```python
from build123d import *

# Parameters (mm, degrees)
EXTRUDE001_DEPTH = 3
FILLET_R         = 1
SKETCH_W         = 40
SKETCH_H         = 40
EXTRUDE_DEPTH    = 140
SKETCH008_R      = 1
EXTRUDE007_DEPTH = 10
EXTRUDE006_DEPTH = 5
EXTRUDE005_DEPTH = 5


with BuildPart() as fillet_body:
    # Sketch001 → Extrude001 (new body)
    with BuildSketch(Plane.XY.offset(-140)):
        with BuildLine():
            Line((0, -2), (40, -2))
            ThreePointArc((40, -2), (41.414214, -1.414214), (42, 0))
            Line((42, 0), (42, 40))
            ThreePointArc((42, 40), (41.414214, 41.414214), (40, 42))
            Line((40, 42), (0, 42))
            ThreePointArc((0, 42), (-1.414214, 41.414214), (-2, 40))
            Line((-2, 40), (-2, 0))
            ThreePointArc((-2, 0), (-1.414214, -1.414214), (0, -2))
        make_face()
    extrude(amount=-EXTRUDE001_DEPTH)

    # Fillet
    fillet_edges = [fillet_body.edges().sort_by_distance(p)[0] for p in [
        (20, 42, -143),
        (-1.414214, 41.414214, -143),
        (-2, 20, -143),
    ]]
    fillet(fillet_edges, radius=FILLET_R)


with BuildPart() as fusion:
    # Sketch → Extrude (new body)
    with BuildSketch(Plane.XY):
        with BuildLine():
            Line((0, -2), (40, -2))
            ThreePointArc((40, -2), (41.414214, -1.414214), (42, 0))
            Line((42, 0), (42, 40))
            ThreePointArc((42, 40), (41.414214, 41.414214), (40, 42))
            Line((40, 42), (0, 42))
            ThreePointArc((0, 42), (-1.414214, 41.414214), (-2, 40))
            Line((-2, 40), (-2, 0))
            ThreePointArc((-2, 0), (-1.414214, -1.414214), (0, -2))
        make_face()
        with Locations((20, 20)):
            Rectangle(SKETCH_W, SKETCH_H, mode=Mode.SUBTRACT)
    extrude(amount=-EXTRUDE_DEPTH)

    # Fusion: union Fillet body
    add(fillet_body.part)


with BuildPart() as extrude007:
    # Sketch008 → Extrude007 (new body)
    with BuildSketch(Plane.XY):
        with Locations((2, 38)):
            Circle(SKETCH008_R)
        with Locations((38, 38)):
            Circle(SKETCH008_R)
        with Locations((20, 2)):
            Circle(SKETCH008_R)
    extrude(amount=-EXTRUDE007_DEPTH)


with BuildPart() as extrude006:
    # Sketch010 → Extrude006 (new body)
    with BuildSketch(Plane.YZ.offset(17.5)):
        Polygon((0, 0), (5, 0), (0, -10), align=None)
    extrude(amount=EXTRUDE006_DEPTH)


with BuildPart() as fusion004:
    # Sketch009 → Extrude005 (new body)
    with BuildSketch(Plane.XZ.offset(-40)):
        Polygon((0, 0), (5, 0), (0, -10), align=None)
        Polygon((40, 0), (35, 0), (40, -10), align=None)
    extrude(amount=EXTRUDE005_DEPTH)

    # Fusion003: union Extrude006
    add(extrude006.part)

    # Cut: cut Extrude007
    add(extrude007.part, mode=Mode.SUBTRACT)


with BuildPart() as fusion004_1:
    # Cut placement: moved
    add(fusion004.part.moved(Location((0, 0, -2))))

    # Fusion004: union Fusion
    add(fusion.part)


solid = fusion004_1.part
```
Could you check a few things on this model? Use its own coordinates, in mm. A direction names the side the tool comes from. Coordinates: 2 decimals unless noted, no trailing zeros. Order: outer loops, then holes, each group sorted by start corner. A loop starts at its lowest first (then second) coordinate and runs counter-clockwise, first axis right, second up. Notation, with made-up numbers: M -35.75,68.25 L 13.25,68.25 A27 cw 13.25,95.25 Z; hole C 37,78 d5. An arc over 180 degrees is marked long. Use a Markdown table: item, result. Add a question column.
Q1. I'm going to push flat-ended pins straight in: pin 1 (3 mm diameter, centred on x = 28, y = 22, fed in from +Z); pin 2 (20 mm diameter, centred on x = 28, y = 29.5, fed in from +Z). Where does each tip first touch, or does it pass through?
Q2. Which directions (+Z, -Z, +X, -X, +Y, -Y) give clear straight access to the entire face, cutting with the end or side of a thin tool? Please do faces 1 (the flat face through (2.535, 36.979, -6.93)), 2 (the flat face through (20, -2, -70)), 3 (the flat face through (3, 37, -2)).
Q3. I want a section at B-B on z = -94.5. List the corners of the cut face in (x, y) for me, then the cut area to 3 significant figures.
Q4. If I drill on L1, parallel to Y at x = 38, z = -5.5; L2, parallel to X at y = 38, z = -7; L3, parallel to Y at x = 11, z = -88, over which ranges is the centre line in solid material (lowest first)?
Q5. I want a section at A-A on y = 19. List the corners of the cut face in (x, z) for me, then the cut area to 3 significant figures.
Q6. We'd pull the mould along X, two halves only. Please class faces 4 (the flat face through (18.854, 2.535, -6.93)), 5 (the flat face through (-2, 20, -70)), 6 (the flat face through (20, 42, -70)): pulls with the +X half, pulls with the -X half, needs draft (parallel to the pull), parting line crosses it, or undercut.
Checked values:
| question | item | result |
|---|---|---|
| 1 | pin 1 | z = -140 |
| 1 | pin 2 | z = -2 |
| 2 | face 1 | none |
| 2 | face 2 | +Z, -Z, +X, -X, -Y |
| 2 | face 3 | +Z |
| 3 | outline | M -2,0 A2 ccw 0,-2 L 40,-2 A2 ccw 42,0 L 42,40 A2 ccw 40,42 L 0,42 A2 ccw -2,40 Z; hole M 0,0 L 40,0 L 40,40 L 0,40 Z |
| 3 | area | 333 mm² |
| 4 | L1 | -2 to 0, 35 to 37, 39 to 42 |
| 4 | L2 | -2 to 1, 39 to 42 |
| 4 | L3 | -2 to 0, 40 to 42 |
| 5 | outline | M -2,-142 A1 ccw -1,-143 L 41,-143 A1 ccw 42,-142 L 42,0 L 40,0 L 40,-140 L 0,-140 L 0,0 L -2,0 Z |
| 5 | area | 692 mm² |
| 6 | face 4 | undercut |
| 6 | face 5 | pulls with the -X half |
| 6 | face 6 | needs draft |
